```python
from build123d import *

# Parameters (mm, degrees)
F1_DEPTH = 50.8
F3_DEPTH = 254


with BuildPart() as f1:
    # F0 (on Front) → F1 (new body)
    with BuildSketch(Plane.XZ):
        Polygon((189.078076, 0), (163.678076, 0), (163.678076, -50.8), (316.078076, -50.8), (316.078076, -12.7), (265.278076, -12.7), (239.878068, 0), (214.478076, 0), (214.478076, -12.7), (227.178076, -12.7), (227.178076, -25.4), (176.378076, -25.4), (176.378076, -12.7), (189.078076, -12.7), align=None)
    extrude(amount=F1_DEPTH)

    # F2 (on Right) → F3 (cut)
    with BuildSketch(Plane.YZ):
        Polygon((-42.799003, -42.036999), (-37.211001, -49.911), (-11.811001, -49.911), (-7.239001, -42.036999), align=None)
    extrude(amount=-F3_DEPTH, mode=Mode.SUBTRACT)


solid = f1.part
```
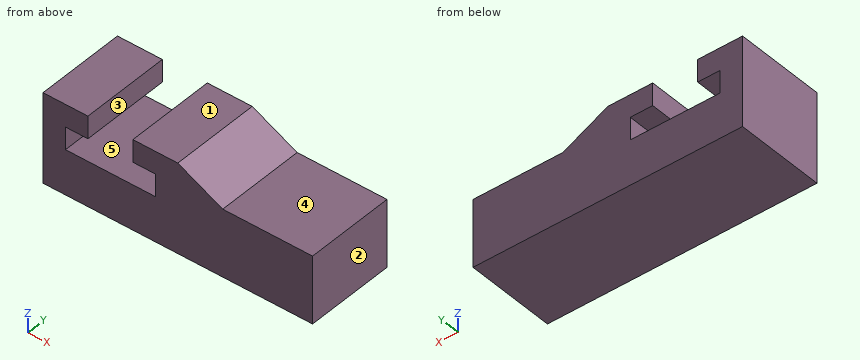
Could you check a few things on this model? Use its own coordinates, in mm. Face numbers are marked on the shaded views. A direction names the side the tool comes from. Give positions to 0.01 mm unless a question says otherwise; leave off trailing zeros. Order: outer loops, then holes, each group sorted by start corner. A loop starts at its lowest first (then second) coordinate and runs counter-clockwise, first axis right, second up.
Q1. Suppose I cut it at B-B, the plane y = -14.5. Write out the boundary of the cut face in (x, z).
Q2. I'm going to push flat-ended pins straight in: P1, Ø1, axis at x = 249.5, y = -5, coming from the +Z side; P2, Ø6.5, axis at y = -13, z = -6, coming from the +X side; P3, Ø15, axis at x = 300.5, y = -22, coming from the +Z side. Where does each tip first touch, or does it pass through?
Q3. Suppose I cut it at A-A, the plane z = -16. Write out the boundary of the cut face in (x, y), and give its area (3 significant figures).
Q4. For the marked faces 1, 2, 3, 4 and 5, which set-ups out of +Z, -Z, +X, -X, +Y, -Y let a thin tool reach every point of the face, with its end or its side?
Q5. Suppose I cut it at C-C, the plane z = -3.5. Write out the boundary of the cut face in (x, y), and give its area (3 significant figures).
Q6. Suppose I cut it at D-D, the plane x = 274.5. Write out the boundary of the cut face in (y, z).
Q7. If I drill on line 1 along X through (y, z) = (-41, -13.5); line 2 along Z through (x, y) = (222, -11.5); line 3 along Z through (x, y) = (302, -6), over which ranges is the centre line in solid material (lowest first)?
Solution:
1. outline: (163.68, -50.8) - (316.08, -50.8) - (316.08, -12.7) - (265.28, -12.7) - (239.88, 0) - (214.48, 0) - (214.48, -12.7) - (227.18, -12.7) - (227.18, -25.4) - (176.38, -25.4) - (176.38, -12.7) - (189.08, -12.7) - (189.08, 0) - (163.68, 0) - close
2. P1: stops at z = -4.56
2. P2: stops at x = 258.38
2. P3: stops at z = -12.7
3. outline: (163.68, -50.8) - (176.38, -50.8) - (176.38, 0) - (163.68, 0) - close; (227.18, -50.8) - (316.08, -50.8) - (316.08, 0) - (227.18, 0) - close
3. area: 5,160 mm2
4. face 1: +Z, +X, -X, +Y, -Y
4. face 2: +Z, -Z, +X, +Y, -Y
4. face 3: +Z, +Y, -Y
4. face 4: +Z, +X, +Y, -Y
4. face 5: +Y, -Y
5. outline: (163.68, -50.8) - (189.08, -50.8) - (189.08, 0) - (163.68, 0) - close; (214.48, -50.8) - (246.88, -50.8) - (246.88, 0) - (214.48, 0) - close
5. area: 2,940 mm2
6. outline: (-50.8, -50.8) - (0, -50.8) - (0, -12.7) - (-50.8, -12.7) - close
7. line 1: x = 163.68 to 176.38, 227.18 to 316.08
7. line 2: z = -50.8 to -25.4, -12.7 to 0
7. line 3: z = -50.8 to -12.7
